```python
from build123d import *

# Parameters (mm, degrees)
EXTRUDE_1_DEPTH     = 36
SKETCH_2_R          = 1.65
CUT_EXTRUDE_1_DEPTH = 38.094473982


with BuildPart() as part:
    # 草图1 → 凸台-拉伸1 (new, symmetric)
    with BuildSketch(Plane.XY):
        Polygon((0, 0), (0, 3), (-4, 3), (-4, -4), (8, -4), (8, 0), align=None)
    extrude(amount=EXTRUDE_1_DEPTH, both=True)

    # 草图2 → 切除-拉伸1 (cut, through all)
    with BuildSketch(Plane(origin=(0, 0, 0), x_dir=(1, 0, 0), z_dir=(0, 1, 0))):
        with Locations(Location((4, 20, 0), (0, 0, 270))):
            Circle(SKETCH_2_R)
        with Locations(Location((4, -20, 0), (0, 0, 90))):
            Circle(SKETCH_2_R)
    extrude(amount=-CUT_EXTRUDE_1_DEPTH, mode=Mode.SUBTRACT)

    # 边界1: read off the stored shape, not the designer's step
    # 边界1: loft between two sections, ruled curve by curve
    other_1_from = [
        Edge.make_line((-34, -54, -73), (-34, -54, -67)),
        Edge.make_line((-34, -54, -67), (-28, -54, -67)),
        Edge.make_line((-28, -54, -67), (-28, -54, -73)),
        Edge.make_line((-28, -54, -73), (-34, -54, -73)),
    ]
    other_1_to = [
        Edge.make_line((-4, -4, -36), (-4, -4, -24)),
        Edge.make_line((-4, -4, -24), (8, -4, -24)),
        Edge.make_line((8, -4, -24), (8, -4, -36)),
        Edge.make_line((8, -4, -36), (-4, -4, -36)),
    ]
    other_1 = Solid(Shell([*[Face.make_surface_from_curves(other_1_from[k], other_1_to[k]) for k in range(4)], Face(Wire(other_1_from)), Face(Wire(other_1_to))]))
    add(other_1)

    # 镜向2: 边界1 across plane
    add(other_1.mirror(Plane.XY))


solid = part.part
```
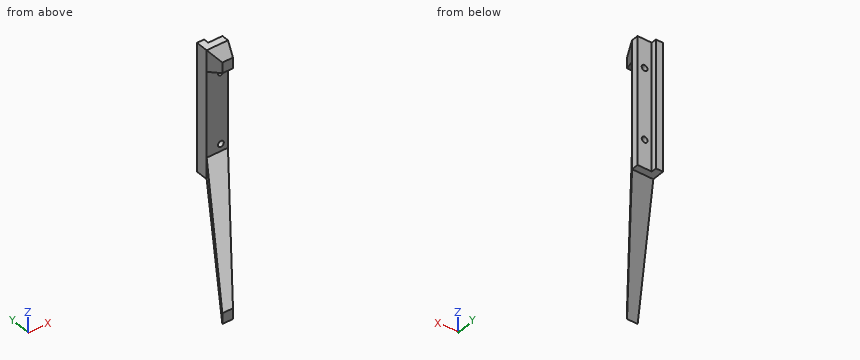
Design review of the part built by this model. Coordinates are the model's own, in mm. Coordinates: 2 decimals unless noted, no trailing zeros. Loops run counter-clockwise (first coordinate to the right, second up) from the corner with the lowest first, then second, coordinate; pieces in that order, holes last.
Q1. We need section A-A on z = 20. State the section outline as (x, y) points, and give its area (3 significant figures).
Reported:
outline: (-4, -4) - (2.35, -4) - (2.35, 0) - (0, 0) - (0, 3) - (-4, 3) - close; (5.65, -4) - (8, -4) - (8, 0) - (5.65, 0) - close
area: 46.8 mm2
Q2. We need section B-B on x = 4. State how many separate pieces and enclosed holes the cut face has, and give its area (3 significant figures).
Reported:
separate pieces: 3
enclosed holes: 0
area: 391 mm2
Q3. For pin 1 (5.5 mm diameter, centred on y = 1, z = 10, fed in from -X); pin 2 (12 mm diameter, centred on x = -12.5, z = -32, fed in from -Y); pin 3 (2 mm diameter, centred on x = -21, z = 52.5, fed in from -Y), all flat-tipped, find the tip position at first contact; note any pin that passes through.
Reported:
pin 1: stops at x = -4
pin 2: stops at y = -20.28
pin 3: stops at y = -38.3
Q4. To check wall thickness, follow line 1 (X direction, y = -2.8, z = 20); line 2 (Z direction, x = -15, y = -33.5); line 3 (Y direction, x = -3, z = -20.5). State the ranges of each line that lie inside material, in increasing order.
Reported:
line 1: x = -4 to 2.35, 5.65 to 8
line 2: z = -57.83 to -49.37, 49.37 to 57.83
line 3: y = -4 to 3
